Geometry check sheet. Reference: the model listing, model coordinates, mm. Face numbers are marked on the shaded views. A direction names the side the tool comes from. Round coordinates to 2 decimals unless told otherwise and drop trailing zeros. Loops run counter-clockwise (first coordinate to the right, second up) from the corner with the lowest first, then second, coordinate; pieces in that order, holes last. Notation, with made-up numbers: (86, 30.5) -> (130, 30.5) arc R12 cw to (130, 34.5) -> close; hole circle Ø9 at (32.5, -10.75). An arc over 180 degrees is marked (long way). Use a Markdown table: item, result. Add a question column.
Q1. Gauge pin test, flat end, axial feed: P1, Ø6, axis at y = 58, z = 37.5, coming from the -X side. Record the tip position at first contact, or that the pin passes through.
Q2. Release check for a two-part mould opening along Y. For the marked faces 1, 2 and 3 record: released by +Y, released by -Y, zero draft, split by the parting line, or undercut.
Q3. Sectioned sample at A-A, the plane y = 40. Enter the section's corners in (x, z).
Q4. Sectioned sample at B-B, the plane x = -42.5. Enter the section's corners in (y, z), then the cut area to 3 significant figures.
Q5. Sectioned sample at C-C, the plane x = -20. Give the number of separate pieces and of enclosed holes in the cut face, then the cut area to 3 significant figures.
Q6. Set-up check for the marked faces 4, 5, 6, 7 and 8: record each of +Z, -Z, +X, -X, +Y, -Y from which the full face is reachable in a straight line by a thin tool's end or side.
Q7. Sectioned sample at D-D, the plane z = 30. Enter the section's corners in (x, y), then the cut area to 3 significant figures.
Q8. Material ranges on L1, parallel to Y at x = -35, z = 4.5; L2, parallel to Z at x = -26.5, y = 72; L3, parallel to Y at x = -6.5, z = 5, recorded low to high.
```python
from build123d import *

# Parameters (mm, degrees)
BOSS_EXTRUDE1_DEPTH = 60
SKETCH2_W           = 115
SKETCH2_H           = 45
CUT_EXTRUDE1_DEPTH  = 81
SKETCH3_W           = 7.5
SKETCH3_H           = 10
BOSS_EXTRUDE2_DEPTH = 10
CHAMFER1_SIZE       = 5
SKETCH4_R           = 2.5
CUT_EXTRUDE2_DEPTH  = 61
CHAMFER2_SIZE       = 10
SKETCH5_R           = 20
CUT_EXTRUDE3_DEPTH  = 76
SKETCH6_R           = 2.5
CUT_EXTRUDE4_DEPTH  = 76
SKETCH7_R           = 4
SKETCH7_R_2         = 2.5
BOSS_EXTRUDE3_DEPTH = 5
SKETCH8_R           = 4
CUT_EXTRUDE5_DEPTH  = 69


with BuildPart() as part:
    # Sketch1 → Boss-Extrude1 (new body)
    with BuildSketch(Plane.XY):
        Polygon((0, 0), (25, 14.43375673), (25, 65.56624327), (0, 80), (-40, 80), (-40, 70), (0, 70), (18, 59.607695155), (18, 20.392304845), (0, 10), (-40, 10), (-40, 0), align=None)
    extrude(amount=BOSS_EXTRUDE1_DEPTH)

    # Sketch2 → Cut-Extrude1 (cut, through all)
    with BuildSketch(Plane(origin=(0, 80, 0), x_dir=(1, 0, 0), z_dir=(0, 1, 0))):
        with Locations((-40, -30)):
            Rectangle(SKETCH2_W, SKETCH2_H)
    extrude(amount=-CUT_EXTRUDE1_DEPTH, mode=Mode.SUBTRACT)

    # Sketch3 → Boss-Extrude2 (add)
    with BuildSketch(Plane.ZY.offset(40)):
        with Locations((3.75, 75)):
            Rectangle(SKETCH3_W, SKETCH3_H)
        with Locations((56.25, 75)):
            Rectangle(SKETCH3_W, SKETCH3_H)
        with Locations((56.25, 5)):
            Rectangle(SKETCH3_W, SKETCH3_H)
        with Locations((3.75, 5)):
            Rectangle(SKETCH3_W, SKETCH3_H)
    extrude(amount=BOSS_EXTRUDE2_DEPTH)

    # Chamfer1
    chamfer1_edges = [part.edges().sort_by_distance(p)[0] for p in [
        (-50, 5, 52.5),
        (-50, 5, 7.5),
        (-50, 75, 7.5),
        (-50, 75, 52.5),
    ]]
    chamfer(chamfer1_edges, length=CHAMFER1_SIZE)

    # Sketch4 → Cut-Extrude2 (cut, through all)
    with BuildSketch(Plane(origin=(0, 0, 0), x_dir=(-1, 0, 0), z_dir=(0, 0, -1))):
        with Locations((20, 75)):
            Circle(SKETCH4_R)
        with Locations((35, 75)):
            Circle(SKETCH4_R)
        with Locations((35, 5)):
            Circle(SKETCH4_R)
        with Locations((20, 5)):
            Circle(SKETCH4_R)
    extrude(amount=-CUT_EXTRUDE2_DEPTH, mode=Mode.SUBTRACT)

    # Chamfer2
    chamfer2_edges = [part.edges().sort_by_distance(p)[0] for p in [
        (17.5, 15.103629711, 7.5),
        (17.5, 64.896370289, 7.5),
        (17.5, 15.103629711, 52.5),
        (17.5, 64.896370289, 52.5),
    ]]
    chamfer(chamfer2_edges, length=CHAMFER2_SIZE)

    # Sketch5 → Cut-Extrude3 (cut, through all)
    with BuildSketch(Plane(origin=(25, 0, 0), x_dir=(0, 0, -1), z_dir=(1, 0, 0))):
        with Locations((-30, 40)):
            Circle(SKETCH5_R)
    extrude(amount=-CUT_EXTRUDE3_DEPTH, mode=Mode.SUBTRACT)

    # Sketch6 → Cut-Extrude4 (cut, through all)
    with BuildSketch(Plane(origin=(25, 0, 0), x_dir=(0, 0, -1), z_dir=(1, 0, 0))):
        with Locations((-53.55, 63.55)):
            Circle(SKETCH6_R)
        with Locations((-6.45, 63.55)):
            Circle(SKETCH6_R)
        with Locations((-6.45, 16.45)):
            Circle(SKETCH6_R)
        with Locations((-53.55, 16.45)):
            Circle(SKETCH6_R)
    extrude(amount=-CUT_EXTRUDE4_DEPTH, mode=Mode.SUBTRACT)

    # Sketch7 → Boss-Extrude3 (add)
    with BuildSketch(Plane(origin=(25, 0, 0), x_dir=(0, 0, -1), z_dir=(1, 0, 0))):
        with Locations((-53.55, 63.55)):
            Circle(SKETCH7_R)
        with Locations((-53.55, 63.55)):
            Circle(SKETCH7_R_2, mode=Mode.SUBTRACT)
        with Locations((-6.45, 63.55)):
            Circle(SKETCH7_R)
        with Locations((-6.45, 63.55)):
            Circle(SKETCH7_R_2, mode=Mode.SUBTRACT)
        with Locations((-6.45, 16.45)):
            Circle(SKETCH7_R)
        with Locations((-6.45, 16.45)):
            Circle(SKETCH7_R_2, mode=Mode.SUBTRACT)
        with Locations((-53.55, 16.45)):
            Circle(SKETCH7_R)
        with Locations((-53.55, 16.45)):
            Circle(SKETCH7_R_2, mode=Mode.SUBTRACT)
    extrude(amount=-BOSS_EXTRUDE3_DEPTH)

    # Sketch8 → Cut-Extrude5 (cut, through all)
    with BuildSketch(Plane.ZY.offset(-18)):
        with Locations((6.45, 63.55)):
            Circle(SKETCH8_R)
        with Locations((53.55, 63.55)):
            Circle(SKETCH8_R)
        with Locations((53.55, 16.45)):
            Circle(SKETCH8_R)
        with Locations((6.45, 16.45)):
            Circle(SKETCH8_R)
    extrude(amount=CUT_EXTRUDE5_DEPTH, mode=Mode.SUBTRACT)


solid = part.part
```
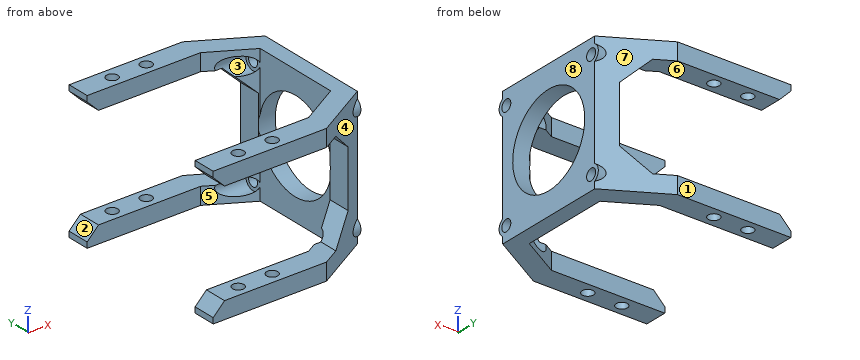
Values:
| question | item | result |
|---|---|---|
| 1 | P1 | x = 17.5 |
| 2 | face 1 | released by +Y |
| 2 | face 2 | zero draft |
| 2 | face 3 | undercut |
| 3 | outline | (18, 0) -> (25, 0) -> (25, 10) -> (18, 10) -> close; (18, 50) -> (25, 50) -> (25, 60) -> (18, 60) -> close |
| 4 | outline | (0, 0) -> (10, 0) -> (10, 7.5) -> (0, 7.5) -> close; (0, 52.5) -> (10, 52.5) -> (10, 60) -> (0, 60) -> close; (70, 0) -> (80, 0) -> (80, 7.5) -> (70, 7.5) -> close; (70, 52.5) -> (80, 52.5) -> (80, 60) -> (70, 60) -> close |
| 4 | area | 300 mm^2 |
| 5 | separate pieces | 8 |
| 5 | enclosed holes | 0 |
| 5 | area | 150 mm^2 |
| 6 | face 4 | +X, -Y |
| 6 | face 5 | +Z, -Z, -X |
| 6 | face 6 | -X, +Y, -Y |
| 6 | face 7 | +X, +Y |
| 6 | face 8 | +Z, -Z, +X, +Y, -Y |
| 7 | outline | (17.5, 10.1) -> (25, 14.43) -> (25, 20) -> (17.5, 20) -> close; (17.5, 60) -> (25, 60) -> (25, 65.57) -> (17.5, 69.9) -> close |
| 7 | area | 116 mm^2 |
| 8 | L1 | 0 to 2.5, 7.5 to 10, 70 to 72.5, 77.5 to 80 |
| 8 | L2 | 0 to 7.5, 52.5 to 60 |
| 8 | L3 | 0 to 10, 70 to 80 |
